```python
from build123d import *

# Parameters (mm, degrees)
SKETCH_1_W             = 102
SKETCH_1_H             = 80
EXTRUDE_1_DEPTH        = 4
SKETCH_5_R             = 1.505
EXTRUDE_3_DEPTH        = 3
SKETCH_16_W            = 10
SKETCH_16_H            = 4.3
EXTRUDE_6_DEPTH        = 37.5
FILLET_3_R             = 1
SKETCH_17_R            = 1.05
SKETCH_17_R_2          = 0.95
CUT_EXTRUDE_10_DEPTH   = 12.5
SKETCH_18_W            = 102
SKETCH_18_H            = 10
CUT_EXTRUDE_11_DEPTH   = 12.5
FILLET_3_OF_MIRROR_2_R = 1
SKETCH_21_W            = 5.636629149
SKETCH_21_H            = 7.556578014
CUT_EXTRUDE_14_DEPTH   = 97.037752993
FILLET_7_R             = 2
SKETCH_22_W            = 16.2
SKETCH_22_H            = 26.510678642
CUT_EXTRUDE_15_DEPTH   = 2
SKETCH_23_R            = 1.75
CUT_EXTRUDE_16_DEPTH   = 74.275166389
SKETCH_25_W            = 11
SKETCH_25_H            = 4
SKETCH_25_R            = 1
EXTRUDE_7_DEPTH        = 4
EXTRUDE_START          = 3
SKETCH_27_R            = 1.5
SKETCH_27_R_2          = 1
EXTRUDE_8_DEPTH        = 3
FILLET_8_R             = 1
FILLET_8_OF_MIRROR_7_R = 1
SKETCH_28_W            = 16
SKETCH_28_H            = 32
CUT_EXTRUDE_17_DEPTH   = 10
SKETCH_29_W            = 94
SKETCH_29_H            = 4
EXTRUDE_9_DEPTH        = 10
SKETCH_30_R            = 5
EXTRUDE_10_DEPTH       = 10
SKETCH_31_R            = 3.5
CUT_EXTRUDE_18_DEPTH   = 8
SKETCH_32_R            = 1.75
CUT_EXTRUDE_19_DEPTH   = 8


with BuildPart() as part:
    # 草图1 → 凸台-拉伸1 (new body)
    with BuildSketch(Plane(origin=(0, 0, 0), x_dir=(1, 0, 0), z_dir=(0, 1, 0))):
        Rectangle(SKETCH_1_W, SKETCH_1_H)
    extrude(amount=EXTRUDE_1_DEPTH)

    # 草图5 → 凸台-拉伸3 (add)
    with BuildSketch(Plane(origin=(44, 0, 0), x_dir=(0, 0, -1), z_dir=(1, 0, 0))):
        with BuildLine():
            Line((-28.004232899, 10.2), (-28.004232899, 4))
            Line((-28.004232899, 4), (-21.995767101, 4))
            Line((-21.995767101, 4), (-21.995767101, 10.2))
            ThreePointArc((-21.995767101, 10.2), (-25, 13.204232899), (-28.004232899, 10.2))
        make_face()
        with Locations((-25, 10.2)):
            Circle(SKETCH_5_R, mode=Mode.SUBTRACT)
    extrude_3 = extrude(amount=EXTRUDE_3_DEPTH)

    # 镜向1: 凸台-拉伸3 across plane
    add(extrude_3.mirror(Plane(origin=(0, 0, 0), x_dir=(0, 0, 1), z_dir=(1, 0, 0))))

    # 草图16 → 凸台-拉伸6 (add)
    with BuildSketch(Plane(origin=(0, 4, 0), x_dir=(1, 0, 0), z_dir=(0, 1, 0))):
        with Locations((34.66, -4.250125)):
            Rectangle(SKETCH_16_W, SKETCH_16_H)
        with Locations((34.66, 23.349875)):
            Rectangle(SKETCH_16_W, SKETCH_16_H)
    extrude_6 = extrude(amount=EXTRUDE_6_DEPTH)

    # 圆角3
    fillet_3_edges = [part.edges().sort_by_distance(p)[0] for p in [
        (39.66, 22.75, 2.100125),
        (39.66, 22.75, -21.199875),
    ]]
    fillet(fillet_3_edges, radius=FILLET_3_R)

    # 草图17 → 切除-拉伸10 (cut)
    with BuildSketch(Plane(origin=(39.66, 0, 0), x_dir=(0, 0, -1), z_dir=(1, 0, 0))):
        with Locations((-4.350125, 10.1)):
            Circle(SKETCH_17_R)
        with Locations((23.449875, 10.1)):
            Circle(SKETCH_17_R)
        with Locations((23.449875, 22.3)):
            Circle(SKETCH_17_R_2)
        with Locations((23.449875, 34.5)):
            Circle(SKETCH_17_R_2)
        with Locations((-4.350125, 34.5)):
            Circle(SKETCH_17_R_2)
        with Locations((-4.350125, 22.3)):
            Circle(SKETCH_17_R_2)
    cut_extrude_10 = extrude(amount=-CUT_EXTRUDE_10_DEPTH, mode=Mode.SUBTRACT)

    # 草图18 → 切除-拉伸11 (cut)
    with BuildSketch(Plane(origin=(0, 4, 0), x_dir=(1, 0, 0), z_dir=(0, 1, 0))):
        with Locations((0, -35)):
            Rectangle(SKETCH_18_W, SKETCH_18_H)
    extrude(amount=-CUT_EXTRUDE_11_DEPTH, mode=Mode.SUBTRACT)

    # 镜向2: 凸台-拉伸6, 切除-拉伸10 across plane
    add(extrude_6.mirror(Plane(origin=(0, 0, 0), x_dir=(0, 0, 1), z_dir=(1, 0, 0))))
    add(cut_extrude_10.mirror(Plane(origin=(0, 0, 0), x_dir=(0, 0, 1), z_dir=(1, 0, 0))), mode=Mode.SUBTRACT)

    # 圆角3 of 镜向2
    fillet_3_of_mirror_2_edges = [part.edges().sort_by_distance(p)[0] for p in [
        (-39.66, 22.75, 2.100125),
        (-39.66, 22.75, -21.199875),
    ]]
    fillet(fillet_3_of_mirror_2_edges, radius=FILLET_3_OF_MIRROR_2_R)

    # 草图21 → 切除-拉伸14 (cut, through all)
    with BuildSketch(Plane.XY.offset(30)):
        with Locations((49.818314575, 1.602871311)):
            Rectangle(SKETCH_21_W, SKETCH_21_H)
    cut_extrude_14 = extrude(amount=-CUT_EXTRUDE_14_DEPTH, mode=Mode.SUBTRACT)

    # 镜向5: 切除-拉伸14 across plane
    add(cut_extrude_14.mirror(Plane(origin=(0, 0, 0), x_dir=(0, 0, 1), z_dir=(1, 0, 0))), mode=Mode.SUBTRACT)

    # 圆角7
    fillet_7_edges = [part.edges().sort_by_distance(p)[0] for p in [
        (47, 2, 30),
    ]]
    fillet(fillet_7_edges, radius=FILLET_7_R)

    # 草图22 → 切除-拉伸15 (cut)
    with BuildSketch(Plane(origin=(0, 4, 0), x_dir=(1, 0, 0), z_dir=(0, 1, 0))):
        with Locations((17.79, -16.744660679)):
            Rectangle(SKETCH_22_W, SKETCH_22_H)
    cut_extrude_15 = extrude(amount=-CUT_EXTRUDE_15_DEPTH, mode=Mode.SUBTRACT)

    # 草图23 → 切除-拉伸16 (cut, through all)
    with BuildSketch(Plane(origin=(0, 2, 0), x_dir=(1, 0, 0), z_dir=(0, 1, 0))):
        with Locations(Location((13.89, -7.5, 0), (0, 0, 270))):
            Circle(SKETCH_23_R)
        with Locations(Location((21.89, -26, 0), (0, 0, 270))):
            Circle(SKETCH_23_R)
    cut_extrude_16 = extrude(amount=-CUT_EXTRUDE_16_DEPTH, mode=Mode.SUBTRACT)

    # 镜向6: 切除-拉伸15, 切除-拉伸16 across plane
    add(cut_extrude_15.mirror(Plane(origin=(0, 0, 0), x_dir=(0, 0, 1), z_dir=(1, 0, 0))), mode=Mode.SUBTRACT)
    add(cut_extrude_16.mirror(Plane(origin=(0, 0, 0), x_dir=(0, 0, 1), z_dir=(1, 0, 0))), mode=Mode.SUBTRACT)

    # 草图25 → 凸台-拉伸7 (add)
    with BuildSketch(Plane.XY.offset(30)):
        with Locations((-35.5, 6)):
            Rectangle(SKETCH_25_W, SKETCH_25_H)
        with Locations((-38, 5.5)):
            Circle(SKETCH_25_R, mode=Mode.SUBTRACT)
        with Locations((-33, 5.5)):
            Circle(SKETCH_25_R, mode=Mode.SUBTRACT)
    extrude_7 = extrude(amount=-EXTRUDE_7_DEPTH)

    # 草图27 → 凸台-拉伸8 (add)
    # profile 1 of 2: a face of its own
    with BuildSketch(Plane.XY.offset(30).offset(EXTRUDE_START)):
        with Locations(Location((-38, 5.5, 0), (0, 0, 180))):
            Circle(SKETCH_27_R)
        with Locations((-38, 5.5)):
            Circle(SKETCH_27_R_2, mode=Mode.SUBTRACT)
    # profile 2 of 2: a face of its own
    with BuildSketch(Plane.XY.offset(30).offset(EXTRUDE_START)):
        with Locations(Location((-33, 5.5, 0), (0, 0, 180))):
            Circle(SKETCH_27_R)
        with Locations((-33, 5.5)):
            Circle(SKETCH_27_R_2, mode=Mode.SUBTRACT)
    extrude_8 = extrude(amount=-EXTRUDE_8_DEPTH)

    # 圆角8
    fillet_8_edges = [part.edges().sort_by_distance(p)[0] for p in [
        (-35.5, 8, 26),
    ]]
    fillet(fillet_8_edges, radius=FILLET_8_R)

    # 镜向7: 凸台-拉伸7, 凸台-拉伸8 across plane
    add(extrude_7.mirror(Plane(origin=(0, 0, 0), x_dir=(0, 0, 1), z_dir=(1, 0, 0))))
    add(extrude_8.mirror(Plane(origin=(0, 0, 0), x_dir=(0, 0, 1), z_dir=(1, 0, 0))))

    # 圆角8 of 镜向7
    fillet_8_of_mirror_7_edges = [part.edges().sort_by_distance(p)[0] for p in [
        (35.5, 8, 26),
    ]]
    fillet(fillet_8_of_mirror_7_edges, radius=FILLET_8_OF_MIRROR_7_R)

    # 草图28 → 切除-拉伸17 (cut)
    with BuildSketch(Plane.XZ):
        with Locations((0, 14)):
            Rectangle(SKETCH_28_W, SKETCH_28_H)
    extrude(amount=-CUT_EXTRUDE_17_DEPTH, mode=Mode.SUBTRACT)

    # 草图29 → 凸台-拉伸9 (add)
    with BuildSketch(Plane(origin=(0, 0, -40), x_dir=(-1, 0, 0), z_dir=(0, 0, -1))):
        with Locations((0, 2)):
            Rectangle(SKETCH_29_W, SKETCH_29_H)
    extrude(amount=EXTRUDE_9_DEPTH)

    # 草图30 → 凸台-拉伸10 (add)
    with BuildSketch(Plane.XZ):
        with Locations(Location((-23, -40, 0), (0, 0, 270))):
            Circle(SKETCH_30_R)
        with Locations(Location((0, -40, 0), (0, 0, 270))):
            Circle(SKETCH_30_R)
        with Locations(Location((23, -40, 0), (0, 0, 270))):
            Circle(SKETCH_30_R)
    extrude(amount=-EXTRUDE_10_DEPTH)

    # 草图31 → 切除-拉伸18 (cut)
    with BuildSketch(Plane.XZ):
        with Locations(Location((23, -40, 0), (0, 0, 270))):
            Circle(SKETCH_31_R)
        with Locations(Location((-23, -40, 0), (0, 0, 270))):
            Circle(SKETCH_31_R)
        with Locations(Location((0, -40, 0), (0, 0, 270))):
            Circle(SKETCH_31_R)
    extrude(amount=-CUT_EXTRUDE_18_DEPTH, mode=Mode.SUBTRACT)

    # 草图32 → 切除-拉伸19 (cut)
    with BuildSketch(Plane(origin=(0, 10, 0), x_dir=(1, 0, 0), z_dir=(0, 1, 0))):
        with Locations(Location((0, 40, 0), (0, 0, 270))):
            Circle(SKETCH_32_R)
        with Locations(Location((23, 40, 0), (0, 0, 270))):
            Circle(SKETCH_32_R)
        with Locations(Location((-23, 40, 0), (0, 0, 270))):
            Circle(SKETCH_32_R)
    extrude(amount=-CUT_EXTRUDE_19_DEPTH, mode=Mode.SUBTRACT)


solid = part.part
```
Geometry check sheet. Reference: the model listing, model coordinates, mm. A direction names the side the tool comes from. Coordinates: 2 decimals unless noted, no trailing zeros. Order: outer loops, then holes, each group sorted by start corner. A loop starts at its lowest first (then second) coordinate and runs counter-clockwise, first axis right, second up. Notation, with made-up numbers: M 83,28 L 118,28 A15 ccw 118,35 Z; hole C 46.25,-2.5 d5. An arc over 180 degrees is marked long. Answer as a JSON object with one key per item and string values.
Q1. Cross-section at B-B on z = -40. Give the number of separate pieces and of enclosed holes in the cut face, and give its area (3 significant figures).
Results are:
{"separate pieces": "4", "enclosed holes": "0", "area": "367 mm²"}
Q2. Release check for a two-part mould opening along X. For faces 1 (the flat face through (35, 22, 6.4)), 2 (the flat face through (47, 3.6, -1.8)), 3 (the flat face through (-8, 2, 14)) record: released by +X, released by -X, zero draft, split by the parting line, or undercut.
Results are:
{"face 1": "zero draft", "face 2": "released by +X", "face 3": "undercut"}
Q3. Cross-section at C-C on z = -4. Record the cut outline in (x, y), and give its area (3 significant figures).
Results are:
{"outline": "M -47,0 L 47,0 L 47,4 L -47,4 Z", "area": "376 mm²"}
Q4. Tool access check on faces 4 (the flat face through (8, 2, 14)), 5 (the flat face through (29.66, 22, 3)), 6 (the cylindrical face through (-20.635, 3.944, -37.42)), 7 (the flat face through (-34, 22, -21.2)), 8 (the flat face through (-45, 7, 28.004)). Record the directions out of +Z, -Z, +X, -X, +Y, -Y that give a thin tool (end or side, any length) a straight path to the whole face; none if there is none.
Results are:
{"face 4": "+Z, +Y, -Y", "face 5": "+Z, -Z, +Y", "face 6": "-Y", "face 7": "+X, -X, +Y", "face 8": "+Z, -X, +Y"}
Q5. Cross-section at A-A on z = 15.5. Record the cut outline in (x, y), and give its area (3 significant figures).
Results are:
{"outline": "M -47,0 L -8,0 L -8,4 L -9.69,4 L -9.69,2 L -25.89,2 L -25.89,4 L -47,4 Z; M 8,0 L 47,0 L 47,4 L 25.89,4 L 25.89,2 L 9.69,2 L 9.69,4 L 8,4 Z", "area": "247 mm²"}
Q6. Depth check by flat-ended pin: pin 1 Ø2 at (x, y) = (27.5, 5.5) entering from +Z; pin 2 Ø2 at (x, y) = (29.5, 21.5) entering from -Z; pin 3 Ø3 at (x, y) = (3.5, 2.5) entering from +Z. Enter the tip coordinate at first touch or a pass-through.
Results are:
{"pin 1": "stops at z = -36.43", "pin 2": "stops at z = -25.5", "pin 3": "stops at z = -2"}
Q7. Scan lines: line 1 (X direction, y = 9, z = -40); line 2 (Z direction, x = 35, y = 27); line 3 (X direction, y = 1, z = 7). Record each from-to range of solid material in increasing order.
Results are:
{"line 1": "x = -28 to -24.75, -21.25 to -18, -5 to -1.75, 1.75 to 5, 18 to 21.25, 24.75 to 28", "line 2": "z = -25.5 to -21.2, 2.1 to 6.4", "line 3": "x = -47 to -15.57, -12.21 to -8, 8 to 12.21, 15.57 to 47"}
